```python
from build123d import *

# Parameters (mm, degrees)
SKETCH_1_W          = 59
SKETCH_1_H          = 65
SKETCH_1_W_2        = 55
SKETCH_1_H_2        = 61
EXTRUDE_1_DEPTH     = 25
SKETCH_2_W          = 59
SKETCH_2_H          = 65
EXTRUDE_2_DEPTH     = 2
EXTRUDE_3_DEPTH     = 2
SKETCH_4_R          = 5
CUT_EXTRUDE_1_DEPTH = 71.215738976
SKETCH_5_W          = 5
SKETCH_5_H          = 0.5
REVOLVE_1_ANGLE     = 180
SKETCH_7_W          = 5
SKETCH_7_H          = 0.5
REVOLVE_2_ANGLE     = 180


with BuildPart() as part:
    # Эскиз1 → Бобышка-Вытянуть1 (new body)
    with BuildSketch(Plane(origin=(0, 0, 0), x_dir=(1, 0, 0), z_dir=(0, 1, 0))):
        Rectangle(SKETCH_1_W, SKETCH_1_H)
        Rectangle(SKETCH_1_W_2, SKETCH_1_H_2, mode=Mode.SUBTRACT)
    extrude(amount=EXTRUDE_1_DEPTH)

    # Эскиз2 → Бобышка-Вытянуть2 (add)
    with BuildSketch(Plane.XZ):
        Rectangle(SKETCH_2_W, SKETCH_2_H)
    extrude(amount=EXTRUDE_2_DEPTH)

    # Эскиз3 → Бобышка-Вытянуть3 (add)
    with BuildSketch(Plane(origin=(0, 0, 0), x_dir=(1, 0, 0), z_dir=(0, 1, 0))):
        with BuildLine():
            Line((-27.5, 25.5), (-27.5, 30.5))
            Line((-27.5, 30.5), (-22.5, 30.5))
            ThreePointArc((-22.5, 30.5), (-23.964466094, 26.964466094), (-27.5, 25.5))
        make_face()
        with BuildLine():
            Line((27.5, 30.5), (22.5, 30.5))
            ThreePointArc((22.5, 30.5), (23.964466094, 26.964466094), (27.5, 25.5))
            Line((27.5, 25.5), (27.5, 30.5))
        make_face()
        with BuildLine():
            Line((27.5, -25.5), (27.5, -30.5))
            Line((27.5, -30.5), (22.5, -30.5))
            ThreePointArc((22.5, -30.5), (23.964466094, -26.964466094), (27.5, -25.5))
        make_face()
        with BuildLine():
            Line((-27.5, -25.5), (-27.5, -30.5))
            Line((-27.5, -30.5), (-22.5, -30.5))
            ThreePointArc((-22.5, -30.5), (-23.964466094, -26.964466094), (-27.5, -25.5))
        make_face()
    extrude(amount=EXTRUDE_3_DEPTH)

    # Эскиз4 → Вырез-Вытянуть1 (cut, through all)
    with BuildSketch(Plane.ZY.offset(-27.5)):
        with Locations((17, 10)):
            Circle(SKETCH_4_R)
        with Locations((-18.5, 10)):
            Circle(SKETCH_4_R)
    extrude(amount=-CUT_EXTRUDE_1_DEPTH, mode=Mode.SUBTRACT)

    # Эскиз5 → Повернуть1 (revolve)
    with BuildSketch(Plane(origin=(0, 0, 30.5), x_dir=(-1, 0, 0), z_dir=(0, 0, -1))):
        with Locations((-25, 3.75)):
            Rectangle(SKETCH_5_W, SKETCH_5_H)
        with Locations((25, 3.75)):
            Rectangle(SKETCH_5_W, SKETCH_5_H)
    revolve(axis=Axis((27.5, 4, 30.5), (1, 0, 0)), revolution_arc=REVOLVE_1_ANGLE)

    # Эскиз7 → Повернуть2 (revolve)
    with BuildSketch(Plane.XY.offset(-30.5)):
        with Locations((-25, 3.75)):
            Rectangle(SKETCH_7_W, SKETCH_7_H)
        with Locations((25, 3.75)):
            Rectangle(SKETCH_7_W, SKETCH_7_H)
    revolve(axis=Axis((-27.5, 4, -30.5), (-1, 0, 0)), revolution_arc=REVOLVE_2_ANGLE)


solid = part.part
```
Work out the finished part from the listing and answer in its coordinate system (mm). A direction names the side the tool comes from. Round coordinates to 2 decimals unless told otherwise and drop trailing zeros. Loops run counter-clockwise (first coordinate to the right, second up) from the corner with the lowest first, then second, coordinate; pieces in that order, holes last.
(1) The mould has two halves that part along X. Classify faces 4 (the flat face through (0, 0, 0)), 5 (the flat face through (0, 12, -32.5)), 6 (the flat face through (-29.5, 12, 0)): pulls with the +X half, pulls with the -X half, needs draft (parallel to the pull), parting line crosses it, or undercut.
Computed values:
face 4: undercut
face 5: needs draft
face 6: pulls with the -X half
(2) The part is cut by section C-C, the plane x = -9.5. Give the vertices of the cut face in (y, z).
Computed values:
outline: (-2, -32.5) - (25, -32.5) - (25, -30.5) - (0, -30.5) - (0, 30.5) - (25, 30.5) - (25, 32.5) - (-2, 32.5) - close
(3) The part is cut by section A-A, the plane z = -18.5. Give the vertices of the cut face in (x, y), and give its area (3 significant figures).
Computed values:
outline: (-29.5, -2) - (29.5, -2) - (29.5, 5) - (27.5, 5) - (27.5, 0) - (-27.5, 0) - (-27.5, 25) - (-29.5, 25) - close; (27.5, 15) - (29.5, 15) - (29.5, 25) - (27.5, 25) - close
area: 198 mm2
(4) The part is cut by section B-B, the plane y = 10. Give the vertices of the cut face in (x, z), and give its area (3 significant figures).
Computed values:
outline: (-29.5, -32.5) - (29.5, -32.5) - (29.5, -23.5) - (27.5, -23.5) - (27.5, -30.5) - (-27.5, -30.5) - (-27.5, 30.5) - (27.5, 30.5) - (27.5, 22) - (29.5, 22) - (29.5, 32.5) - (-29.5, 32.5) - close; (27.5, -13.5) - (29.5, -13.5) - (29.5, 12) - (27.5, 12) - close
area: 440 mm2
(5) The part is cut by section D-D, the plane z = -9. Give the vertices of the cut face in (x, y), and give its area (3 significant figures).
Computed values:
outline: (-29.5, -2) - (29.5, -2) - (29.5, 25) - (27.5, 25) - (27.5, 0) - (-27.5, 0) - (-27.5, 25) - (-29.5, 25) - close
area: 218 mm2
(6) For faces 1 (the flat face through (26, 2, -29)), 2 (the flat face through (0, 12, 32.5)), 3 (the cylindrical face through (28.49, 11.5, 21.77)), determine the directions among +Z, -Z, +X, -X, +Y, -Y from which every point of the face is accessible in a straight line to the end or side of a thin tool.
Computed values:
face 1: none
face 2: +Z, +X, -X, +Y, -Y
face 3: +X
(7) Each of these flat-tipped pins is pushed along its axis until it touches: P1, Ø5.5, axis at x = 24, z = -27.5, coming from the +Y side; P2, Ø16.5, axis at x = -7.5, z = -4, coming from the +Y side; P3, Ø1.5, axis at x = 25.5, z = 29, coming from the +Y side. Where does it stop, or does it pass through?
Computed values:
P1: stops at y = 4.43
P2: stops at y = 0
P3: stops at y = 2
(8) Find the intervals of material crossed by L1, parallel to X at y = 5.75, z = 1; L2, parallel to Z at x = -9.5, y = 18.75; L3, parallel to Y at x = 26.5, z = -22, in increasing order.
Computed values:
L1: x = -29.5 to -27.5, 27.5 to 29.5
L2: z = -32.5 to -30.5, 30.5 to 32.5
L3: y = -2 to 0
